Here's how the part is built. I have some questions about the finished solid (model axes, mm). A direction names the side the tool comes from. Coordinates: 2 decimals unless noted, no trailing zeros. Order: outer loops, then holes, each group sorted by start corner. A loop starts at its lowest first (then second) coordinate and runs counter-clockwise, first axis right, second up. Notation, with made-up numbers: (24.25, -33) - (83.25, -33) arc R11 cw to (83.25, -23) - close; hole circle Ø1 at (19, 13.25). An arc over 180 degrees is marked (long way). Answer as CSV lines item,"result". Start each with the question number.
Item 1: Imagine slicing it at A-A on z = 28.5. List the corners of the cut face in (x, y) for me.
Item 2: I need wall thicknesses on line 1 (Y direction, x = -19, z = 33); line 2 (X direction, y = -17, z = 12); line 3 (Z direction, x = -26.5, y = 12.5). Which ranges of each line are inside material? Lowest first, please.
Item 3: Imagine slicing it at B-B on y = -19.5. List the corners of the cut face in (x, z) for me.
Item 4: We'd pull the mould along Y, two halves only. Please class faces 3 (the face through (-1, -25, 31)), 4 (the face through (-1, 0, 2)), 5 (the face through (-40, 0, 31)): pulls with the +Y half, pulls with the -Y half, needs draft (parallel to the pull), parting line crosses it, or undercut.
Item 5: I'm going to push a flat-ended pin straight in: pin 1 (3 mm diameter, centred on x = 15, y = 10, fed in from +Z). Where does the tip first touch, or does it pass through?
Item 6: Imagine slicing it at C-C on x = 4.5. List the corners of the cut face in (y, z) for me, and give its area (3 significant figures).
Item 7: On a 3-axis mill with a long thin cutter (end or side, diameter ignored), from which of +Z, -Z, +X, -X, +Y, -Y can I reach the whole of each face in a straight line? I mean faces 1 (the face through (-1, -22, 32)), 2 (the face through (0, -24, 62)). Say none if no direction works.
from build123d import *

# Parameters (mm, degrees)
F0_W     = 80
F0_H     = 50
F1_DEPTH = 2
F2_W     = 80
F2_H     = 50
F2_W_2   = 74
F2_H_2   = 44
F3_DEPTH = 60


with BuildPart() as f1:
    # F0 (on Top) → F1 (new body)
    with BuildSketch(Plane.XY):
        Rectangle(F0_W, F0_H)
    extrude(amount=F1_DEPTH)

    # F2 (on face) → F3 (join)
    with BuildSketch(Plane.XY.offset(2)):
        Rectangle(F2_W, F2_H)
        Rectangle(F2_W_2, F2_H_2, mode=Mode.SUBTRACT)
    extrude(amount=F3_DEPTH)


solid = f1.part
Responses:
1,outline,"(-40, -25) - (40, -25) - (40, 25) - (-40, 25) - close; hole (-37, -22) - (37, -22) - (37, 22) - (-37, 22) - close"
2,line 1,"y = -25 to -22, 22 to 25"
2,line 2,"x = -40 to -37, 37 to 40"
2,line 3,"z = 0 to 2"
3,outline,"(-40, 0) - (40, 0) - (40, 62) - (37, 62) - (37, 2) - (-37, 2) - (-37, 62) - (-40, 62) - close"
4,face 3,"pulls with the -Y half"
4,face 4,"undercut"
4,face 5,"needs draft"
5,pin 1,"stops at z = 2"
6,outline,"(-25, 0) - (25, 0) - (25, 62) - (22, 62) - (22, 2) - (-22, 2) - (-22, 62) - (-25, 62) - close"
6,area,"460 mm^2"
7,face 1,"+Z"
7,face 2,"+Z, +X, -X, +Y, -Y"
